Geometry check sheet. Reference: drawing and pictorial views, mm from the part's lowest x, y, z. Coordinates: 2 decimals unless noted, no trailing zeros. Write each loop counter-clockwise with the first axis right and the second up, starting at its lowest first coordinate (ties: lowest second). Pieces come first, ordered by that corner, then holes. Notation, with made-up numbers: (7.25, -37.75) -> (22.25, -37.75) arc R23 cw to (22.25, -24.75) -> close; hole circle Ø3 at (15, 58). An arc over 180 degrees is marked (long way). Use a Markdown table: item, result. Add a question column.
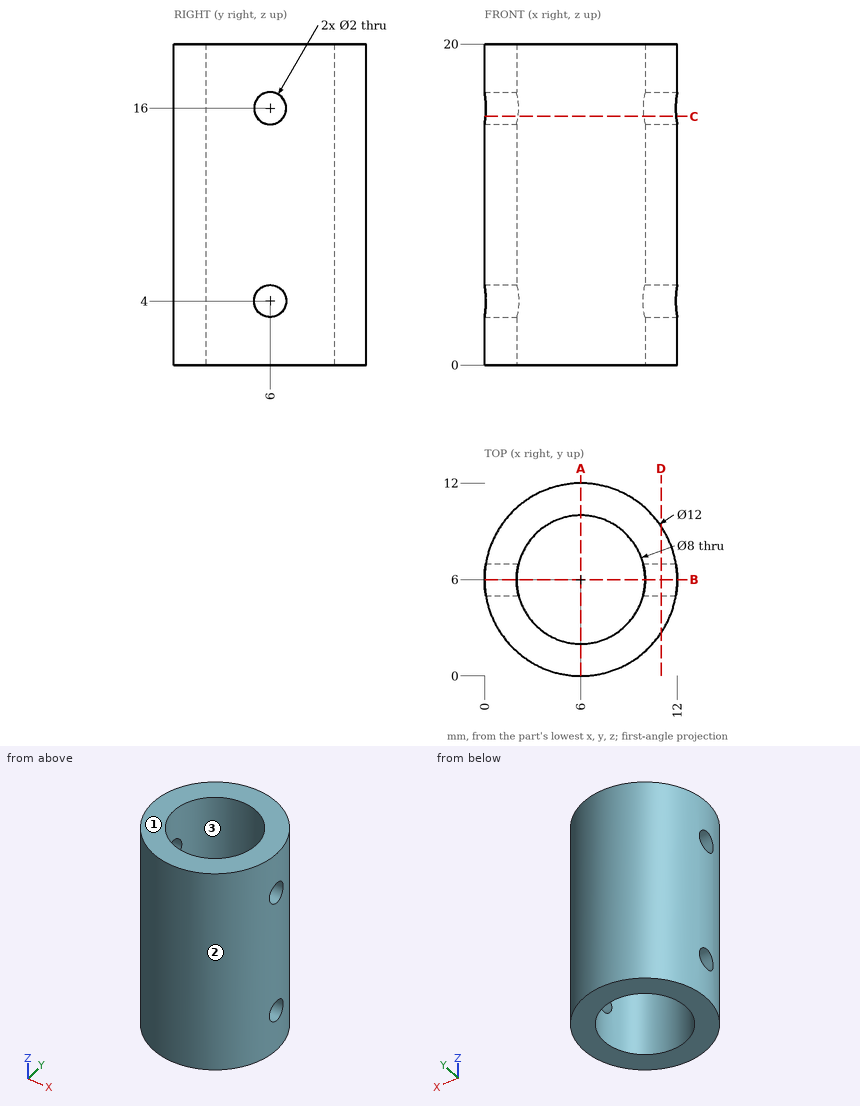
1) Cross-section at C-C on z = 15.5. Record the boundary of the cut face in (x, y).
2) Release check for a two-part mould opening along X. For the marked faces 1, 2 and 3 record: released by +X, released by -X, zero draft, split by the parting line, or undercut.
3) Thickness scan on L1, parallel to Y at x = 6, z = 10.25; L2, parallel to X at y = 8.5, z = 9.75; L3, parallel to X at y = 3, z = 15.75. Record the ranges inside material, lowest first.
4) Cross-section at D-D on x = 11. Record the boundary of the cut face in (y, z), then the cut area to 3 significant figures.
5) Gauge pin test, flat ends, axial feed: pin 1 (5 mm diameter, centred on x = 9.5, z = 10.5, fed in from +Y); pin 2 (3 mm diameter, centred on y = 3.5, z = 7, fed in from -X); pin 3 (2 mm diameter, centred on x = 9, z = 8, fed in from +Y). Record the tip position at first contact, or that the pin passes through.
6) Cross-section at A-A on x = 6. Record the boundary of the cut face in (y, z).
7) Cross-section at B-B on y = 6. Record the boundary of the cut face in (x, z), then the cut area to 3 significant figures.
Returned:
| question | item | result |
|---|---|---|
| 1 | outline | (0.06, 5.13) arc R6 ccw to (11.94, 5.13) -> (9.91, 5.13) arc R4 cw to (2.09, 5.13) -> close; (0.06, 6.87) -> (2.09, 6.87) arc R4 cw to (9.91, 6.87) -> (11.94, 6.87) arc R6 ccw to start |
| 2 | face 1 | zero draft |
| 2 | face 2 | split by the parting line |
| 2 | face 3 | undercut |
| 3 | L1 | y = 0 to 2, 10 to 12 |
| 3 | L2 | x = 0.55 to 2.88, 9.12 to 11.45 |
| 3 | L3 | x = 0.8 to 3.35, 8.65 to 11.2 |
| 4 | outline | (2.68, 0) -> (9.32, 0) -> (9.32, 20) -> (2.68, 20) -> close; hole circle Ø2 at (6, 4); hole circle Ø2 at (6, 16) |
| 4 | area | 126 mm² |
| 5 | pin 1 | stops at y = 11.92 |
| 5 | pin 2 | stops at x = 0.08 |
| 5 | pin 3 | stops at y = 11.66 |
| 6 | outline | (0, 0) -> (2, 0) -> (2, 20) -> (0, 20) -> close; (10, 0) -> (12, 0) -> (12, 20) -> (10, 20) -> close |
| 7 | outline | (0, 0) -> (2, 0) -> (2, 3) -> (0, 3) -> close; (0, 5) -> (2, 5) -> (2, 15) -> (0, 15) -> close; (0, 17) -> (2, 17) -> (2, 20) -> (0, 20) -> close; (10, 0) -> (12, 0) -> (12, 3) -> (10, 3) -> close; (10, 5) -> (12, 5) -> (12, 15) -> (10, 15) -> close; (10, 17) -> (12, 17) -> (12, 20) -> (10, 20) -> close |
| 7 | area | 64.0 mm² |
